The model under review builds one solid part; all positions refer to its coordinate system, in mm. Coordinates: 2 decimals unless noted, no trailing zeros. Loops run counter-clockwise (first coordinate to the right, second up) from the corner with the lowest first, then second, coordinate; pieces in that order, holes last. Notation, with made-up numbers: M 83,-18 L 102,-18 A26 ccw 102,0 Z; hole C 43,-40 d5. An arc over 180 degrees is marked long. Return JSON: item names as keys, results as strings.
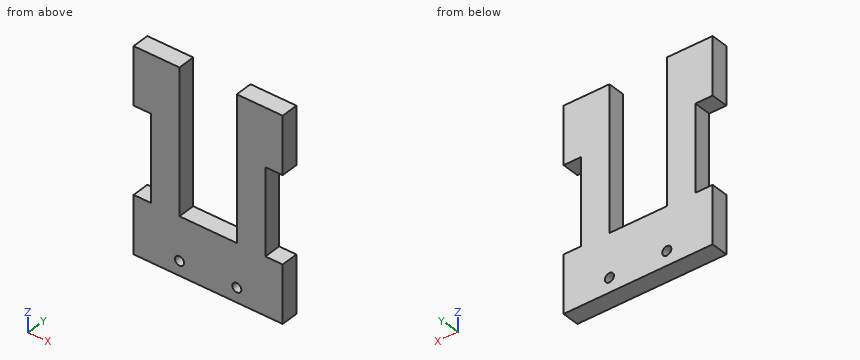
```python
from build123d import *

# Parameters (mm, degrees)
BOSS_EXTRUDE1_DEPTH = 6
SKETCH2_R           = 1.5875
CUT_EXTRUDE1_DEPTH  = 45.011362169


with BuildPart() as part:
    # Sketch1 → Boss-Extrude1 (new body)
    with BuildSketch(Plane(origin=(0, 0, 0), x_dir=(1, 0, 0), z_dir=(0, 1, 0))):
        Polygon((-10, -35), (-10, 15), (10, 15), (10, -35), (26, -35), (26, -15), (20, -15), (20, 15), (26, 15), (26, 35), (-26, 35), (-26, 15), (-20, 15), (-20, -15), (-26, -15), (-26, -35), align=None)
    extrude(amount=BOSS_EXTRUDE1_DEPTH)

    # Sketch2 → Cut-Extrude1 (cut, through all)
    with BuildSketch(Plane(origin=(0, 6, 0), x_dir=(1, 0, 0), z_dir=(0, 1, 0))):
        with Locations(Location((-10, 30, 0), (0, 0, 270))):
            Circle(SKETCH2_R)
        with Locations(Location((10, 30, 0), (0, 0, 90))):
            Circle(SKETCH2_R)
    extrude(amount=-CUT_EXTRUDE1_DEPTH, mode=Mode.SUBTRACT)


solid = part.part
```
1. To check wall thickness, follow line 1 (X direction, y = 3.2, z = -30); line 2 (Z direction, x = -21, y = 4.9); line 3 (X direction, y = 3, z = -13). State the ranges of each line that lie inside material, in increasing order.
Check values:
{"line 1": "-26 to -11.59, -8.41 to 8.41, 11.59 to 26", "line 2": "-35 to -15, 15 to 35", "line 3": "-20 to -10, 10 to 20"}
2. Add section D-D on x = -2.5. Give the boundary of the cut face in (y, z), plus the area to 3 significant figures.
Check values:
{"outline": "M 0,-35 L 6,-35 L 6,-15 L 0,-15 Z", "area": "120 mm²"}
3. Add section C-C on y = 1.7. Give the boundary of the cut face in (x, z) (1 decimal), plus the area to 3 significant figures.
Check values:
{"outline": "M -26,-35 L 26,-35 L 26,-15 L 20,-15 L 20,15 L 26,15 L 26,35 L 10,35 L 10,-15 L -10,-15 L -10,35 L -26,35 L -26,15 L -20,15 L -20,-15 L -26,-15 Z; hole C -10,-30 d3.2; hole C 10,-30 d3.2", "area": "2,260 mm²"}
4. Add section B-B on z = 2. Give the boundary of the cut face in (x, y).
Check values:
{"outline": "M -20,0 L -10,0 L -10,6 L -20,6 Z; M 10,0 L 20,0 L 20,6 L 10,6 Z"}
5. Add section A-A on z = -30. Give the boundary of the cut face in (x, y), plus the area to 3 significant figures.
Check values:
{"outline": "M -26,0 L -11.59,0 L -11.59,6 L -26,6 Z; M -8.41,0 L 8.41,0 L 8.41,6 L -8.41,6 Z; M 11.59,0 L 26,0 L 26,6 L 11.59,6 Z", "area": "274 mm²"}
6. Insertion check: pin 1 Ø3 at (y, z) = (4, 11) entering from +X; pin 2 Ø3 at (y, z) = (3, 12) entering from -X; pin 3 Ø2 at (x, y) = (-2, 4) entering from +Z. Each pin has a flat end and moves straight along its axis. Give the tip position at first contact, or say it passes through.
Check values:
{"pin 1": "x = 20", "pin 2": "x = -20", "pin 3": "z = -15"}
